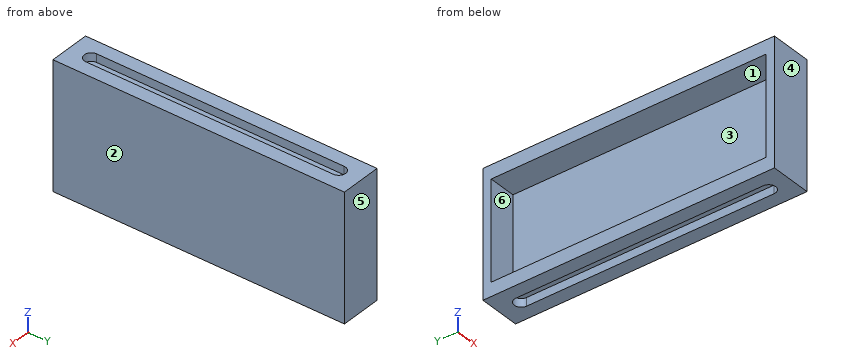
from build123d import *

# Parameters (mm, degrees)
SKETCH4_W           = 15
SKETCH4_H           = 100
BOSS_EXTRUDE1_DEPTH = 5
SKETCH5_W           = 36
SKETCH5_H           = 100
BOSS_EXTRUDE2_DEPTH = 5
CUT_EXTRUDE1_DEPTH  = 3
SKETCH7_W           = 15
SKETCH7_H           = 46
BOSS_EXTRUDE3_DEPTH = 3


with BuildPart() as part:
    # Sketch4 → Boss-Extrude1 (new body)
    with BuildSketch(Plane.XY):
        Rectangle(SKETCH4_W, SKETCH4_H)
    boss_extrude1 = extrude(amount=BOSS_EXTRUDE1_DEPTH)

    # Sketch5 → Boss-Extrude2 (add)
    with BuildSketch(Plane(origin=(7.5, 0, 0), x_dir=(0, 0, -1), z_dir=(1, 0, 0))):
        with Locations((18, 0)):
            Rectangle(SKETCH5_W, SKETCH5_H)
    extrude(amount=-BOSS_EXTRUDE2_DEPTH)

    # Mirror1: Boss-Extrude1 across plane
    add(boss_extrude1.mirror(Plane.XY.offset(-18)))

    # Sketch6 → Cut-Extrude1 (cut)
    with BuildSketch(Plane.XY.offset(5)):
        with BuildLine():
            Line((2.5, 45), (2.5, -45))
            ThreePointArc((2.5, -45), (0, -47.5), (-2.5, -45))
            Line((-2.5, -45), (-2.5, 45))
            ThreePointArc((-2.5, 45), (0, 47.5), (2.5, 45))
        make_face()
    cut_extrude1 = extrude(amount=-CUT_EXTRUDE1_DEPTH, mode=Mode.SUBTRACT)

    # Mirror2: Cut-Extrude1 across plane
    add(cut_extrude1.mirror(Plane.XY.offset(-18)), mode=Mode.SUBTRACT)

    # Sketch7 → Boss-Extrude3 (add)
    with BuildSketch(Plane.XZ.offset(50)):
        with Locations((0, -18)):
            Rectangle(SKETCH7_W, SKETCH7_H)
    boss_extrude3 = extrude(amount=BOSS_EXTRUDE3_DEPTH)

    # Mirror3: Boss-Extrude3 across plane
    add(boss_extrude3.mirror(Plane.ZX))


solid = part.part
Input: part model. Units: mm. Frame: model coordinates. Face numbers are marked on the shaded views. A direction names the side the tool comes from. Coordinates: 2 decimals unless noted, no trailing zeros. Loops run counter-clockwise (first coordinate to the right, second up) from the corner with the lowest first, then second, coordinate; pieces in that order, holes last.
(1) Set-up query: the marked faces 5 and 6. Return all of +Z, -Z, +X, -X, +Y, -Y with unobstructed straight access to the full face (end or side cutting, diameter ignored); none if empty.
(2) Pull-direction query (Y, two-part tool) for the marked faces 1, 2, 3 and 4; classes: released by +Y, released by -Y, zero draft, split by the parting line, or undercut.
(3) Section C-C on z = -25. Return the cut outline in (x, y).
(4) Material intervals for probe 1 along Z at (x, y) = (-1.5, 17); probe 2 along Y at (x, z) = (2, -27.5); probe 3 along Z at (x, y) = (-3, 33), sorted ascending.
(5) Section A-A on x = -1.5. Return the cut outline in (y, z).
(6) First-contact query: pin 1 Ø18 at (y, z) = (4.5, -22) entering from -X; pin 2 Ø2.5 at (x, y) = (0, -22) entering from +Z. Flat tips, straight axial feed; report the tip coordinate or a pass-through.
(7) Section B-B on y = 4.5. Return the cut outline in (x, z), then the cut area to 3 significant figures.
Data:
1. face 5: +Z, -Z, +X, -X, +Y
1. face 6: -X
2. face 1: undercut
2. face 2: zero draft
2. face 3: undercut
2. face 4: released by -Y
3. outline: (-7.5, -53) - (7.5, -53) - (7.5, 53) - (-7.5, 53) - (-7.5, 50) - (2.5, 50) - (2.5, -50) - (-7.5, -50) - close
4. probe 1: z = -38 to -36, 0 to 2
4. probe 2: y = -53 to -50, 50 to 53
4. probe 3: z = -41 to -36, 0 to 5
5. outline: (-53, -41) - (-47, -41) - (-47, -38) - (47, -38) - (47, -41) - (53, -41) - (53, 5) - (47, 5) - (47, 2) - (-47, 2) - (-47, 5) - (-53, 5) - close; hole (-50, -36) - (50, -36) - (50, 0) - (-50, 0) - close
6. pin 1: stops at x = 2.5
6. pin 2: stops at z = 2
7. outline: (-7.5, -41) - (-2.5, -41) - (-2.5, -38) - (2.5, -38) - (2.5, -41) - (7.5, -41) - (7.5, 5) - (2.5, 5) - (2.5, 2) - (-2.5, 2) - (-2.5, 5) - (-7.5, 5) - (-7.5, 0) - (2.5, 0) - (2.5, -36) - (-7.5, -36) - close
7. area: 300 mm2
